from build123d import *

# Parameters (mm, degrees)
SKETCH1_R           = 1.25
BOSS_EXTRUDE1_DEPTH = 2.5
BOSS_EXTRUDE2_DEPTH = 2.5
BOSS_EXTRUDE4_START = 2.5
BOSS_EXTRUDE4_DEPTH = 2.5
SKETCH5_W           = 10
SKETCH5_H           = 6
BOSS_EXTRUDE6_DEPTH = 8
CHAMFER1_SIZE       = 2
SKETCH6_R           = 1.6
CUT_EXTRUDE1_DEPTH  = 8
CHAMFER2_SIZE       = 1
CHAMFER3_SIZE       = 1.2
SKETCH7_W           = 2.5
SKETCH7_H           = 22
CUT_EXTRUDE2_DEPTH  = 55.835083878
CHAMFER4_SIZE       = 2


with BuildPart() as part:
    # Sketch1 → Boss-Extrude1 (new body)
    with BuildSketch(Plane(origin=(0, 0, 0), x_dir=(0, 0, -1), z_dir=(1, 0, 0))):
        with BuildLine():
            ThreePointArc((-20.08490506, 22.793126127), (-22.206225403, 21.914446471), (-23.08490506, 19.793126127))
            Line((-23.08490506, 19.793126127), (-23.08490506, -12.206873873))
            ThreePointArc((-23.08490506, -12.206873873), (-22.206225403, -14.328194216), (-20.08490506, -15.206873873))
            Line((-20.08490506, -15.206873873), (11.91509494, -15.206873873))
            ThreePointArc((11.91509494, -15.206873873), (14.036415284, -14.328194216), (14.91509494, -12.206873873))
            Line((14.91509494, -12.206873873), (14.91509494, 19.793126127))
            ThreePointArc((14.91509494, 19.793126127), (14.036415284, 21.914446471), (11.91509494, 22.793126127))
            Line((11.91509494, 22.793126127), (-20.08490506, 22.793126127))
        make_face()
        with Locations((-19.08490506, -11.206873873)):
            Circle(SKETCH1_R, mode=Mode.SUBTRACT)
        with Locations((10.91509494, -11.206873873)):
            Circle(SKETCH1_R, mode=Mode.SUBTRACT)
        with BuildLine():
            ThreePointArc((-19.08490506, 17.543126127), (-19.968788536, 19.677009604), (-17.83490506, 18.793126127))
            ThreePointArc((-17.83490506, 18.793126127), (-18.201021583, 17.909242651), (-19.08490506, 17.543126127))
        make_face(mode=Mode.SUBTRACT)
        with BuildLine():
            Line((-19.08490506, -8.206873873), (-19.08490506, 15.793126127))
            ThreePointArc((-19.08490506, 15.793126127), (-16.963584716, 16.671805784), (-16.08490506, 18.793126127))
            Line((-16.08490506, 18.793126127), (7.91509494, 18.793126127))
            ThreePointArc((7.91509494, 18.793126127), (8.793774597, 16.671805784), (10.91509494, 15.793126127))
            Line((10.91509494, 15.793126127), (10.91509494, -8.206873873))
            ThreePointArc((10.91509494, -8.206873873), (8.793774597, -9.085553529), (7.91509494, -11.206873873))
            Line((7.91509494, -11.206873873), (-16.08490506, -11.206873873))
            ThreePointArc((-16.08490506, -11.206873873), (-16.963584716, -9.085553529), (-19.08490506, -8.206873873))
        make_face(mode=Mode.SUBTRACT)
        with Locations((10.91509494, 18.793126127)):
            Circle(SKETCH1_R, mode=Mode.SUBTRACT)
    extrude(amount=BOSS_EXTRUDE1_DEPTH)

    # Sketch2 → Boss-Extrude2 (add)
    with BuildSketch(Plane.ZY):
        with BuildLine():
            Line((-17.11509494, 19.793126127), (-17.11509494, -12.206873873))
            ThreePointArc((-17.11509494, -12.206873873), (-15.592050202, -15.883829135), (-11.91509494, -17.406873873))
            Line((-11.91509494, -17.406873873), (20.08490506, -17.406873873))
            ThreePointArc((20.08490506, -17.406873873), (23.761860322, -15.883829135), (25.28490506, -12.206873873))
            Line((25.28490506, -12.206873873), (25.28490506, 19.793126127))
            ThreePointArc((25.28490506, 19.793126127), (23.761860322, 23.470081389), (20.08490506, 24.993126127))
            Line((20.08490506, 24.993126127), (-11.91509494, 24.993126127))
            ThreePointArc((-11.91509494, 24.993126127), (-15.592050202, 23.470081389), (-17.11509494, 19.793126127))
        make_face()
        with BuildLine():
            Line((-14.91509494, 19.793126127), (-14.91509494, -12.206873873))
            ThreePointArc((-14.91509494, -12.206873873), (-14.036415284, -14.328194216), (-11.91509494, -15.206873873))
            Line((-11.91509494, -15.206873873), (20.08490506, -15.206873873))
            ThreePointArc((20.08490506, -15.206873873), (22.206225403, -14.328194216), (23.08490506, -12.206873873))
            Line((23.08490506, -12.206873873), (23.08490506, 19.793126127))
            ThreePointArc((23.08490506, 19.793126127), (22.206225403, 21.914446471), (20.08490506, 22.793126127))
            Line((20.08490506, 22.793126127), (-11.91509494, 22.793126127))
            ThreePointArc((-11.91509494, 22.793126127), (-14.036415284, 21.914446471), (-14.91509494, 19.793126127))
        make_face(mode=Mode.SUBTRACT)
    extrude(amount=-BOSS_EXTRUDE2_DEPTH)

    # Sketch3 → Boss-Extrude4 (add)
    with BuildSketch(Plane.ZY.offset(BOSS_EXTRUDE4_START)):
        with BuildLine():
            Line((-17.11509494, 19.793126127), (-17.11509494, -12.206873873))
            ThreePointArc((-17.11509494, -12.206873873), (-15.592050202, -15.883829135), (-11.91509494, -17.406873873))
            Line((-11.91509494, -17.406873873), (20.08490506, -17.406873873))
            ThreePointArc((20.08490506, -17.406873873), (23.761860322, -15.883829135), (25.28490506, -12.206873873))
            Line((25.28490506, -12.206873873), (25.28490506, 19.793126127))
            ThreePointArc((25.28490506, 19.793126127), (23.761860322, 23.470081389), (20.08490506, 24.993126127))
            Line((20.08490506, 24.993126127), (-11.91509494, 24.993126127))
            ThreePointArc((-11.91509494, 24.993126127), (-15.592050202, 23.470081389), (-17.11509494, 19.793126127))
        make_face()
        with BuildLine():
            Line((-15.11509494, 19.793126127), (-15.11509494, -12.206873873))
            ThreePointArc((-15.11509494, -12.206873873), (-14.17783664, -14.469615573), (-11.91509494, -15.406873873))
            Line((-11.91509494, -15.406873873), (20.08490506, -15.406873873))
            ThreePointArc((20.08490506, -15.406873873), (22.34764676, -14.469615573), (23.28490506, -12.206873873))
            Line((23.28490506, -12.206873873), (23.28490506, 19.793126127))
            ThreePointArc((23.28490506, 19.793126127), (22.34764676, 22.055867827), (20.08490506, 22.993126127))
            Line((20.08490506, 22.993126127), (-11.91509494, 22.993126127))
            ThreePointArc((-11.91509494, 22.993126127), (-14.17783664, 22.055867827), (-15.11509494, 19.793126127))
        make_face(mode=Mode.SUBTRACT)
    extrude(amount=-BOSS_EXTRUDE4_DEPTH)

    # Sketch5 → Boss-Extrude6 (add)
    with BuildSketch(Plane.XZ.offset(17.406873873)):
        with Locations((0, 4.08490506)):
            Rectangle(SKETCH5_W, SKETCH5_H)
    extrude(amount=BOSS_EXTRUDE6_DEPTH)

    # Chamfer1
    chamfer1_edges = [part.edges().sort_by_distance(p)[0] for p in [
        (-2.5, -17.406873873, 4.08490506),
        (2.5, -17.406873873, 4.08490506),
    ]]
    chamfer(chamfer1_edges, length=CHAMFER1_SIZE - 0.0001)  # a hair under: the kernel refuses the full size

    # Sketch6 → Cut-Extrude1 (cut)
    with BuildSketch(Plane(origin=(0, 0, 1.08490506), x_dir=(-1, 0, 0), z_dir=(0, 0, -1))):
        with Locations((0, -21.406873873)):
            Circle(SKETCH6_R)
    extrude(amount=-CUT_EXTRUDE1_DEPTH, mode=Mode.SUBTRACT)

    # Chamfer2
    chamfer2_edges = [part.edges().sort_by_distance(p)[0] for p in [
        (-5, -25.406873873, 4.08490506),
        (5, -25.406873873, 4.08490506),
    ]]
    chamfer(chamfer2_edges, length=CHAMFER2_SIZE)

    # Chamfer3
    chamfer3_edges = [part.edges().sort_by_distance(p)[0] for p in [
        (0, -25.406873873, 1.08490506),
        (0, -25.406873873, 7.08490506),
    ]]
    chamfer(chamfer3_edges, length=CHAMFER3_SIZE)

    # Sketch7 → Cut-Extrude2 (cut, through all)
    with BuildSketch(Plane.XZ.offset(-22.993126127)):
        with Locations((-1.25, 4.08490506)):
            Rectangle(SKETCH7_W, SKETCH7_H)
    extrude(amount=-CUT_EXTRUDE2_DEPTH, mode=Mode.SUBTRACT)

    # Chamfer4
    chamfer4_edges = [part.edges().sort_by_distance(p)[0] for p in [
        (-2.5, 23.993126127, -6.91509494),
        (-2.5, 23.993126127, 15.08490506),
    ]]
    chamfer(chamfer4_edges, length=CHAMFER4_SIZE)


solid = part.part
The model under review builds one solid part; all positions refer to its coordinate system, in mm. A direction names the side the tool comes from. Round coordinates to 2 decimals unless told otherwise and drop trailing zeros. Write each loop counter-clockwise with the first axis right and the second up, starting at its lowest first coordinate (ties: lowest second). Pieces come first, ordered by that corner, then holes. Notation, with made-up numbers: M 89,6.5 L 124,6.5 A34 cw 124,37.5 Z; hole C 35,45.25 d2. An arc over 180 degrees is marked long. Answer as CSV lines item,"result". Start each with the question number.
Q1. Tool access review of faces 1 (the face through (1, 4, -10.915)), 2 (the face through (-0.07, -24.815, 1.693)), 3 (the face through (-1.3, 22, 22.4)), 4 (the face through (-1.486, 23.979, 16.071)), 5 (the face through (4.507, -24.9, 4.046)): name each direction out of +Z, -Z, +X, -X, +Y, -Y from which nothing blocks a thin tool from reaching the whole face with its end or side.
Q2. The part is to be moulded in two halves that separate along Z. For faces 6 (the face through (1.232, 16.695, -8.771)), 7 (the face through (-0.04, 23.43, 23.8)), 8 (the face through (3.486, -16.393, 4.043)), 9 (the face through (1.232, 19.847, -11.587)), say which applies: +Z half, -Z half, draft (parallel to the pull), parting line (faces both ways), or undercut.
Q3. Clearance check with flat-ended pins moving along their axes: P1, Ø0.6, axis at x = -0.5, y = 23.5, coming from the +Z side; P2, Ø5, axis at y = -14, z = 4.5, coming from the -X side; P3, Ø3, axis at y = 18.79, z = 19.08, coming from the +X side. State where each tip first meets the part, or that it passes through.
Q4. Wall thickness on line 1 along Z through (x, y) = (2, -2); line 2 along Y through (x, z) = (1, 2); line 3 along Z through (x, y) = (-1, -1.5): over which ranges is each line inside the solid? List them lowest first.
Q5. Consider section B-B, the plane z = 10. Give the boundary of the cut face in (x, y), then the cut area to 3 significant figures.
Q6. Consider section A-A, the plane y = 14. Give the boundary of the cut face in (x, z), then the cut area to 3 significant figures.
Q7. Consider section C-C, the plane z = -13. Give the boundary of the cut face in (x, y), then the cut area to 3 significant figures.
Result set:
1,face 1,"+X, -X"
1,face 2,"-Z, +X, -X, -Y"
1,face 3,"-X"
1,face 4,"-X, +Y"
1,face 5,"+Z, -Z, +X, -Y"
2,face 6,"undercut"
2,face 7,"+Z half"
2,face 8,"draft"
2,face 9,"undercut"
3,P1,"stops at z = 24.01"
3,P2,"stops at x = -3.59"
3,P3,"stops at x = 2.5"
4,line 1,"z = -17.12 to -10.92, 19.08 to 25.28"
4,line 2,"y = -25.12 to -22.66, -20.16 to -11.21, 18.79 to 24.99"
4,line 3,"z = -17.12 to -15.12, 23.28 to 25.28"
5,outline,"M -2.5,-17.41 L 2.5,-17.41 L 2.5,-11.21 L 0,-11.21 L 0,-15.41 L -2.5,-15.41 Z; M 0,18.79 L 2.5,18.79 L 2.5,24.99 L 0,24.99 Z"
5,area,"36.0 mm²"
6,outline,"M -2.5,-17.12 L 2.5,-17.12 L 2.5,-10.92 L 0,-10.92 L 0,-15.12 L -2.5,-15.12 Z; M -2.5,23.28 L 0,23.28 L 0,19.08 L 2.5,19.08 L 2.5,25.28 L -2.5,25.28 Z"
6,area,"41.0 mm²"
7,outline,"M -2.5,-17.29 L 2.5,-17.29 L 2.5,24.88 L -2.5,24.88 L -2.5,22.8 L 0,22.8 L 0,-15.22 L -2.5,-15.22 Z"
7,area,"116 mm²"
